Verification items for the finished model (mm, model axes). Round coordinates to 2 decimals unless told otherwise and drop trailing zeros. Write each loop counter-clockwise with the first axis right and the second up, starting at its lowest first coordinate (ties: lowest second). Pieces come first, ordered by that corner, then holes. Notation, with made-up numbers: M 84,69 L 143,69 A13 cw 143,82 Z; hole C 48,84 d8. An arc over 180 degrees is marked long. One line per question, with ' | ' between items. Start each with the question number.
Q1. Gauge pin test, flat ends, axial feed: pin 1 (1 mm diameter, centred on y = 5.5, z = 14, fed in from -X); pin 2 (4 mm diameter, centred on y = 0, z = 0, fed in from -X); pin 3 (4 mm diameter, centred on y = -1.5, z = -12.5, fed in from -X). Record the tip position at first contact, or that the pin passes through.
Q2. Cross-section at A-A (y = -3.5). Record the boundary of the cut face in (x, z) (3 decimals), then the cut area to 3 significant figures.
Q3. Thickness scan on line 1 along X through (y, z) = (0.75, -1.5); line 2 along X through (y, z) = (0.5, 2.5); line 3 along X through (y, z) = (8.5, 20). Record the ranges inside material, lowest first. Write a range as from..to.
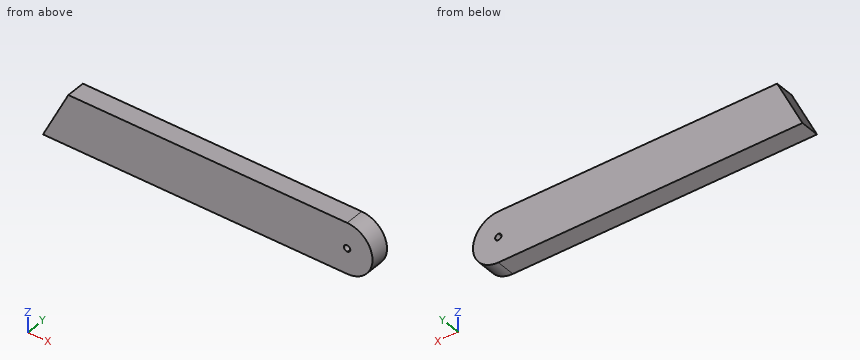
from build123d import *

# Parameters (mm, degrees)
F1_DEPTH = 9.525


with BuildPart() as f1:
    # F0 (on Front) → F1 (new body, symmetric)
    with BuildSketch(Plane.XZ):
        with BuildLine():
            ThreePointArc((139.7, -25.4), (157.6605122421, -17.9605122421), (165.1, 0))
            ThreePointArc((165.1, 0), (157.6605122421, 17.9605122421), (139.7, 25.4))
            Line((139.7, 25.4), (139.7, 3.175))
            ThreePointArc((139.7, 3.175), (141.9450640303, 2.2450640303), (142.875, 0))
            ThreePointArc((142.875, 0), (141.9450640303, -2.2450640303), (139.7, -3.175))
            Line((139.7, -3.175), (139.7, -25.4))
        make_face()
        with BuildLine():
            Line((139.7, 3.175), (139.7, 25.4))
            ThreePointArc((139.7, 25.4), (114.3, 0), (139.7, -25.4))
            Line((139.7, -25.4), (139.7, -3.175))
            ThreePointArc((139.7, -3.175), (136.525, 0), (139.7, 3.175))
        make_face()
        with BuildLine():
            ThreePointArc((139.7, -25.4), (114.3, 0), (139.7, 25.4))
            Line((139.7, 25.4), (-139.7, 25.4))
            Line((-139.7, 25.4), (-139.7, -25.4))
            Line((-139.7, -25.4), (139.7, -25.4))
        make_face()
        Polygon((-139.7, -25.4), (-139.7, 25.4), (-165.1, -25.4), align=None)
    extrude(amount=F1_DEPTH, both=True)


solid = f1.part
Determined:
1) pin 1: stops at x = -145.65 | pin 2: stops at x = -153.4 | pin 3: stops at x = -159.65
2) outline: M -165.1,-25.4 L 139.7,-25.4 A25.4 ccw 139.7,25.4 L -139.7,25.4 Z; hole C 139.7,0 d6.35 | area: 15,800 mm²
3) line 1: x = -153.15..136.9, 142.5..165.06 | line 2: x = -151.15..137.74, 141.66..164.98 | line 3: x = -142.4..155.36
